```python
from build123d import *

# Parameters (mm, degrees)
F1_DEPTH = 4.5
F2_R     = 6
F3_DEPTH = 22
F4_R     = 2
F5_SIZE  = 1


with BuildPart() as f1:
    # F0 (on Top) → F1 (new body)
    with BuildSketch(Plane.XY):
        with BuildLine():
            Line((-8.4913125212, -13.3127669957), (-3.1642680885, -7.8890688591))
            ThreePointArc((-3.1642680885, -7.8890688591), (0, -8.5), (3.1642680885, -7.8890688591))
            Line((3.1642680885, -7.8890688591), (8.4913125212, -13.3127669957))
            ThreePointArc((8.4913125212, -13.3127669957), (9.8181818622, -13.9088228343), (11.1979483169, -13.4482695352))
            ThreePointArc((11.1979483169, -13.4482695352), (15.1554445662, -8.75), (17.2455172129, -2.9735729451))
            ThreePointArc((17.2455172129, -2.9735729451), (16.9544848424, -1.5483834945), (15.7748506735, -0.6973088569))
            Line((15.7748506735, -0.6973088569), (8.4142680885, 1.2041978806))
            ThreePointArc((8.4142680885, 1.2041978806), (7.3612159322, 4.25), (5.25, 6.6848709786))
            Line((5.25, 6.6848709786), (7.2835381524, 14.0100758527))
            ThreePointArc((7.2835381524, 14.0100758527), (7.1363029802, 15.4572063288), (6.047568896, 16.4218424803))
            ThreePointArc((6.047568896, 16.4218424803), (0, 17.5), (-6.047568896, 16.4218424803))
            ThreePointArc((-6.047568896, 16.4218424803), (-7.1363029802, 15.4572063288), (-7.2835381524, 14.0100758527))
            Line((-7.2835381524, 14.0100758527), (-5.25, 6.6848709786))
            ThreePointArc((-5.25, 6.6848709786), (-7.3612159322, 4.25), (-8.4142680885, 1.2041978806))
            Line((-8.4142680885, 1.2041978806), (-15.7748506735, -0.6973088569))
            ThreePointArc((-15.7748506735, -0.6973088569), (-16.9544848424, -1.5483834945), (-17.2455172129, -2.9735729451))
            ThreePointArc((-17.2455172129, -2.9735729451), (-15.1554445662, -8.75), (-11.1979483169, -13.4482695352))
            ThreePointArc((-11.1979483169, -13.4482695352), (-9.8181818622, -13.9088228343), (-8.4913125212, -13.3127669957))
        make_face()
    extrude(amount=F1_DEPTH)

    # F2 (on face) → F3 (join)
    with BuildSketch(Plane.XY.offset(4.5)):
        Circle(F2_R)
        with BuildLine():
            ThreePointArc((2.3, -2.6381811917), (-3.5, 0), (2.3, 2.6381811917))
            Line((2.3, 2.6381811917), (2.3, -2.6381811917))
        make_face(mode=Mode.SUBTRACT)
    extrude(amount=F3_DEPTH)

    # F4
    f4_edges = [f1.edges().sort_by_distance(p)[0] for p in [
        (-6.266769, 10.347473, 0),
        (-12.094559, 0.253445, 0),
        (15.155445, -8.75, 0),
        (7.361216, 4.25, 0),
        (0, -8.5, 0),
        (-7.361216, 4.25, 0),
    ]]
    fillet(f4_edges, radius=F4_R)

    # F5
    f5_edges = [f1.edges().sort_by_distance(p)[0] for p in [
        (-3.5, 0, 26.5),
        (2.3, 0, 26.5),
    ]]
    chamfer(f5_edges, length=F5_SIZE)


solid = f1.part
```
Check sheet for the modelled part. Datum: model origin and axes. Units: mm. A direction names the side the tool comes from. Round coordinates to 2 decimals unless told otherwise and drop trailing zeros. Loops run counter-clockwise (first coordinate to the right, second up) from the corner with the lowest first, then second, coordinate; pieces in that order, holes last. Notation, with made-up numbers: M 62,-12 L 71,-12 A22 cw 71,15 Z; hole C 73,66.5 d1. An arc over 180 degrees is marked long. Answer as a JSON object with one key per item and string values.
1. Mould release check, pull along X, two halves, no side actions. Record for faces 1 (the flat face through (12.15, 0.24, 3.23)), 2 (the flat face through (-5.865, -10.639, 3.232)), 3 (the cylindrical face through (-15.198, -8.675, 3.232)): pulls with the +X half, pulls with the -X half, needs draft (parallel to the pull), parting line crosses it, or undercut.
Reply:
{"face 1": "pulls with the +X half", "face 2": "undercut", "face 3": "pulls with the -X half"}
2. Scan lines: line 1 (Y direction, x = 0, z = 17.75); line 2 (Z direction, x = 13, y = -5); line 3 (Y direction, x = 1, z = 21.25). Record each from-to range of solid material in increasing order.
Reply:
{"line 1": "y = -6 to -3.5, 3.5 to 6", "line 2": "z = 0 to 4.5", "line 3": "y = -5.92 to -3.35, 3.35 to 5.92"}
3. Access from +Z, -Z, +X, -X, +Y, -Y to the whole of each face (thin tool, end or side, straight path). Record for faces 4 (the cylindrical face through (-5.7, -9.61, 0.57)), 5 (the cylindrical face through (11.17, -0.13, 0.57)), 6 (the flat face through (6.253, 10.296, 3.232)), 7 (the cylindrical face through (-7.34, 4.29, 3.23)), 8 (the flat face through (2.8, 0, 26)).
Reply:
{"face 4": "-Z, -Y", "face 5": "-Z, +X, +Y", "face 6": "+Z, -Z, +X", "face 7": "+Z, -Z, -X", "face 8": "+Z"}
4. Section check A-A (x = 0). Record the boundary of the cut face in (y, z).
Reply:
{"outline": "M -8.5,2 A2 ccw -6.5,0 L 15.5,0 A2 ccw 17.5,2 L 17.5,4.5 L 6,4.5 L 6,26.5 L 4.5,26.5 L 3.5,25.5 L 3.5,4.5 L -3.5,4.5 L -3.5,25.5 L -4.5,26.5 L -6,26.5 L -6,4.5 L -8.5,4.5 Z"}
5. Section check B-B (z = 8.25). Record the boundary of the cut face in (x, y).
Reply:
{"outline": "C 0,0 d12; hole M 2.3,-2.64 L 2.3,2.64 A3.5 ccw long Z"}
6. Gauge pin test, flat ends, axial feed: P1, Ø10, axis at x = -4, z = 18.5, coming from the -Y side; P2, Ø12, axis at y = -6, z = 21, coming from the +X side; P3, Ø4.5, axis at x = 0.5, y = 1, coming from the +Z side; P4, Ø1, axis at x = -7, z = 14.5, coming from the -Y side. Record the tip position at first contact, or that the pin passes through.
Reply:
{"P1": "stops at y = -6", "P2": "stops at x = 6", "P3": "stops at z = 25.95", "P4": "passes through"}
